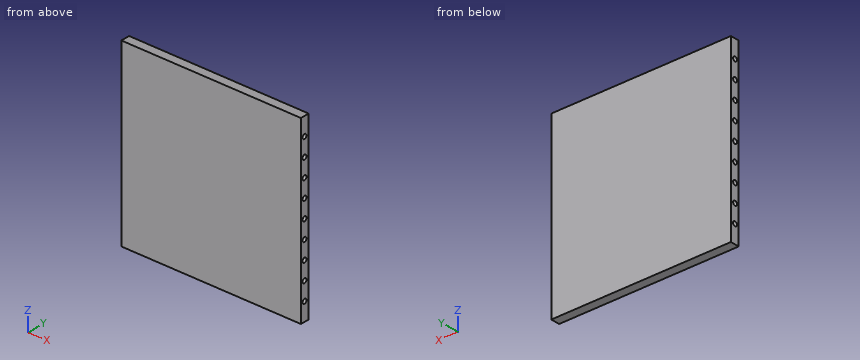
from build123d import *

# Parameters (mm, degrees)
SKETCH1_W           = 127
SKETCH1_H           = 127
BOSS_EXTRUDE1_DEPTH = 6.35
CUT_EXTRUDE1_REACH  = 144.132
SKETCH3_R           = 1.5875
LPATTERN1_COUNT     = 9
LPATTERN1_PITCH     = 12.7


with BuildPart() as part:
    # Sketch1 → Boss-Extrude1 (new body)
    with BuildSketch(Plane(origin=(0, 0, 0), x_dir=(1, 0, 0), z_dir=(0, 1, 0))):
        Rectangle(SKETCH1_W, SKETCH1_H)
    extrude(amount=BOSS_EXTRUDE1_DEPTH)

    # Sketch3 → Cut-Extrude1 (cut, up to next)
    with BuildSketch(Plane.ZY.offset(63.5), mode=Mode.PRIVATE) as cut_extrude1_sk1:
        with Locations((-50.8, 2.973801717)):
            Circle(SKETCH3_R)
    cut_extrude1_tool1 = extrude(cut_extrude1_sk1.sketch, amount=-CUT_EXTRUDE1_REACH, mode=Mode.PRIVATE) & part.part
    cut_extrude1 = cut_extrude1_tool1.solids().sort_by_distance((-63.5, 2.973802, -50.8))[0]
    add(cut_extrude1, mode=Mode.SUBTRACT)

    # LPattern1: Cut-Extrude1 ×9
    with Locations(*[(0, 0, i * LPATTERN1_PITCH) for i in range(1, LPATTERN1_COUNT)]):
        add(cut_extrude1, mode=Mode.SUBTRACT)


solid = part.part
The model under review builds one solid part; all positions refer to its coordinate system, in mm. Round coordinates to 2 decimals unless told otherwise and drop trailing zeros. Write each loop counter-clockwise with the first axis right and the second up, starting at its lowest first coordinate (ties: lowest second). Pieces come first, ordered by that corner, then holes. Notation, with made-up numbers: (-36.75, -10.5) -> (-20.75, -10.5) arc R14 ccw to (-20.75, -3.5) -> close; hole circle Ø6 at (-22, -32). An arc over 180 degrees is marked (long way). Answer as a JSON object with one key per item and string values.
1. We need section A-A on z = 0. State the section outline as (x, y) points.
Results found:
{"outline": "(-63.5, 0) -> (63.5, 0) -> (63.5, 1.39) -> (-63.5, 1.39) -> close; (-63.5, 4.56) -> (63.5, 4.56) -> (63.5, 6.35) -> (-63.5, 6.35) -> close"}
2. We need section B-B on x = -34.5. State how many separate pieces and enclosed holes the cut face has, and give its area (3 significant figures).
Results found:
{"separate pieces": "1", "enclosed holes": "9", "area": "735 mm^2"}
3. To check wall thickness, follow line 1 along Y through (x, z) = (-36, -12.7); line 2 along Y through (x, z) = (22, -25). State the ranges of each line that lie inside material, in increasing order.
Results found:
{"line 1": "y = 0 to 1.39, 4.56 to 6.35", "line 2": "y = 0 to 1.44, 4.51 to 6.35"}
